Autodesk Inventor part; units mm, degrees
ref_plane "YZ Plane" through (0, 0, 0) normal (1, 0, 0) x (0, 1, 0)
ref_plane "XZ Plane" through (0, 0, 0) normal (0, 1, 0) x (-1, 0, 0)
ref_plane "XY Plane" through (0, 0, 0) normal (0, 0, 1) x (1, 0, 0)
sketch "Esboço1" plane through (0, 0, 0) normal (1, 0, 0) x (0, 1, 0)
  line L0 (-504, 129) -> (504, 129)
  line L1 (504, 129) -> (504, -129)
  line L2 (504, -129) -> (-504, -129)
  line L3 (-504, -129) -> (-504, 129)
  line L4 (-504, 129) -> (504, -129) construction
  line L5 (504, 129) -> (-504, -129) construction
  point P0 (0, 0)
  dimension "d0" = 1008
  dimension "d1" = 258
extrude "Extrusão1" add sketch "Esboço1" along normal mid plane 4
sketch "Esboço3" plane through (2, 0, 0) normal (1, 0, 0) x (0, 0, -1)
  line L0 (-133, 630) -> (-125, 630)
  line L1 (-125, 630) -> (-125, 378)
  line L2 (-125, 378) -> (-133, 378)
  line L3 (-133, 378) -> (-133, 630)
  line L4 (129, 504) -> (-129, 504)
  line L5 (-133, 630) -> (-125, 378) construction
  line L6 (-125, 630) -> (-133, 378) construction
  line L7 (-125, 126) -> (-133, 126)
  line L8 (-133, 126) -> (-133, -126)
  line L9 (-133, -126) -> (-125, -126)
  line L10 (-125, -126) -> (-125, 126)
  line L11 (-129, 504) -> (-129, -504)
  line L12 (-125, 126) -> (-133, -126) construction
  line L13 (-133, 126) -> (-125, -126) construction
  line L14 (-125, -378) -> (-133, -378)
  line L15 (-133, -378) -> (-133, -630)
  line L16 (-133, -630) -> (-125, -630)
  line L17 (-125, -630) -> (-125, -378)
  line L18 (-125, -378) -> (-133, -630) construction
  line L19 (-133, -378) -> (-125, -630) construction
  line L20 (125, 630) -> (133, 630)
  line L21 (133, 630) -> (133, 378)
  line L22 (133, 378) -> (125, 378)
  line L23 (125, 378) -> (125, 630)
  line L24 (125, 630) -> (133, 378) construction
  line L25 (133, 630) -> (125, 378) construction
  line L26 (125, 126) -> (133, 126)
  line L27 (133, 126) -> (133, -126)
  line L28 (133, -126) -> (125, -126)
  line L29 (125, -126) -> (125, 126)
  line L30 (129, -504) -> (129, 504)
  line L31 (125, 126) -> (133, -126) construction
  line L32 (133, 126) -> (125, -126) construction
  line L33 (125, -378) -> (133, -378)
  line L34 (133, -378) -> (133, -630)
  line L35 (133, -630) -> (125, -630)
  line L36 (125, -630) -> (125, -378)
  line L37 (125, -378) -> (133, -630) construction
  line L38 (133, -378) -> (125, -630) construction
  point P0 (0, 0)
  point P1 (-129, 0)
  point P2 (-129, -504)
  point P3 (129, 0)
  dimension "d8" = 8
  dimension "d9" = 252
  dimension "d10" = 252
  dimension "d11" = 252
  dimension "d12" = 8
  dimension "d13" = 252
  dimension "d14" = 8
  dimension "d15" = 252
  dimension "d16" = 8
  dimension "d17" = 252
  dimension "d18" = 252
  dimension "d19" = 8
  dimension "d20" = 252
  dimension "d21" = 252
  dimension "d22" = 8
  dimension "d23" = 252
extrude "Extrusão3" cut sketch "Esboço3" along normal through all both and the other way through all
sketch "Esboço4" plane through (2, 0, 0) normal (1, 0, 0) x (0, 0, -1)
  line L0 (-125, 504) -> (125, 504)
  line L1 (-125, 504) -> (-42, 504)
  line L2 (-42, 504) -> (-42, 500)
  line L3 (-42, 500) -> (-125, 500)
  line L4 (-125, 500) -> (-125, 504)
  line L5 (125, 504) -> (42, 504)
  line L6 (42, 504) -> (42, 500)
  line L7 (42, 500) -> (125, 500)
  line L8 (125, 500) -> (125, 504)
  line L9 (-125, -504) -> (125, -504)
  line L10 (-125, -504) -> (-42, -504)
  line L11 (-42, -504) -> (-42, -500)
  line L12 (-42, -500) -> (-125, -500)
  line L13 (-125, -500) -> (-125, -504)
  line L14 (125, -504) -> (42, -504)
  line L15 (42, -504) -> (42, -500)
  line L16 (42, -500) -> (125, -500)
  line L17 (125, -500) -> (125, -504)
  point P0 (0, 0)
  dimension "d26" = 83
  dimension "d27" = 4
  dimension "d28" = 83
  dimension "d29" = 4
  dimension "d30" = 84
  dimension "d31" = 83
  dimension "d32" = 4
  dimension "d33" = 83
  dimension "d34" = 4
  dimension "d35" = 84
extrude "Extrusão4" cut sketch "Esboço4" along normal through all both and the other way through all
sketch "Esboço6" plane through (2, 0, 0) normal (1, 0, 0) x (0, 0, -1)
  point P0 (0, 0)
properties part number "PAREDES LATERAIS"
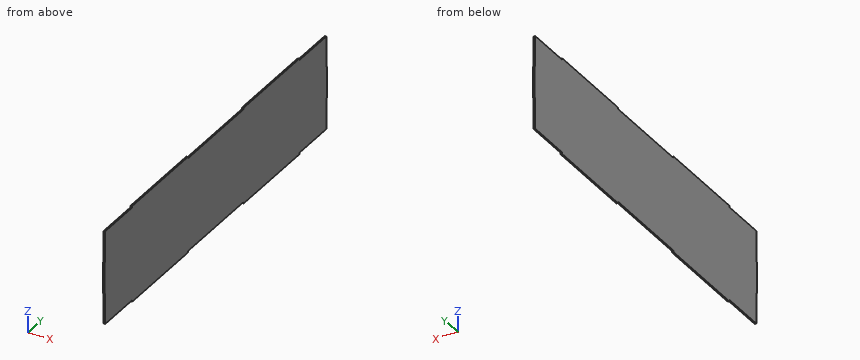
Could you check a few things on this model? Use its own coordinates, in mm. Round coordinates to 2 decimals unless told otherwise and drop trailing zeros. Write each loop counter-clockwise with the first axis right and the second up, starting at its lowest first coordinate (ties: lowest second). Pieces come first, ordered by that corner, then holes. Notation, with made-up numbers: (25.25, 89.5) -> (79.25, 89.5) arc R25 cw to (79.25, 111.5) -> close; hole circle Ø7 at (58, 57). An arc over 180 degrees is marked (long way). Use a Markdown table: item, result.
1. For pin 1 Ø1 at (x, z) = (1, -81) entering from -Y; pin 2 Ø2 at (x, y) = (1, 501.5) entering from -Z; pin 3 Ø2 at (x, z) = (0, 127) entering from +Y, each with a flat end and sliding along its axis, tell me the tip position at first contact or that it passes through.
Answer key:
| item | result |
|---|---|
| pin 1 | stops at y = -500 |
| pin 2 | stops at z = -42 |
| pin 3 | stops at y = 378 |
2. If we section it at A-A (x = 0.4): List the corners of the cut face in (y, z) for me.
Answer key:
| item | result |
|---|---|
| outline | (-504, -42) -> (-500, -42) -> (-500, -125) -> (-378, -125) -> (-378, -129) -> (-126, -129) -> (-126, -125) -> (126, -125) -> (126, -129) -> (378, -129) -> (378, -125) -> (500, -125) -> (500, -42) -> (504, -42) -> (504, 42) -> (500, 42) -> (500, 125) -> (378, 125) -> (378, 129) -> (126, 129) -> (126, 125) -> (-126, 125) -> (-126, 129) -> (-378, 129) -> (-378, 125) -> (-500, 125) -> (-500, 42) -> (-504, 42) -> close |
3. If we section it at B-B (y = 70): List the corners of the cut face in (x, z) for me, then the cut area to 3 significant figures.
Answer key:
| item | result |
|---|---|
| outline | (-2, -125) -> (2, -125) -> (2, 125) -> (-2, 125) -> close |
| area | 1,000 mm^2 |
4. Please list where these lines run through material, in increasing order: probe 1 along Y at (x, z) = (-1.7, -69); probe 2 along Z at (x, y) = (-1.75, -125).
Answer key:
| item | result |
|---|---|
| probe 1 | y = -500 to 500 |
| probe 2 | z = -125 to 125 |
